Could you check a few things on this model? Use its own coordinates, in mm. A direction names the side the tool comes from. Round coordinates to 2 decimals unless told otherwise and drop trailing zeros. Loops run counter-clockwise (first coordinate to the right, second up) from the corner with the lowest first, then second, coordinate; pieces in that order, holes last. Notation, with made-up numbers: (16.25, 17) -> (65.25, 17) arc R11 cw to (65.25, 35) -> close; hole circle Ø5 at (6.5, 69). An arc over 180 degrees is marked (long way). One line per item, written item: value.
```python
from build123d import *
from build123d.topology import SkipClean

# Parameters (mm, degrees)
SKETCH1_R                            = 30
BOSS_EXTRUDE1_DEPTH                  = 4
BOSS_EXTRUDE2_REACH                  = 44.615
BOSS_EXTRUDE2_END_RADIUS             = 30
BOSS_EXTRUDE2_DIRECTION_2_REACH      = 44.615
BOSS_EXTRUDE2_DIRECTION_2_END_RADIUS = 30
SKETCH3_OUTSIDE_W                    = 78.092
SKETCH3_OUTSIDE_H                    = 69.092
SKETCH3_OUTSIDE_R                    = 21.5
CUT_EXTRUDE2_DEPTH                   = 12.5
BOSS_EXTRUDE3_DEPTH                  = 18
BOSS_EXTRUDE4_DEPTH                  = 15
BOSS_EXTRUDE5_DEPTH                  = 15
CUT_EXTRUDE3_DEPTH                   = 44.292609069
CUT_EXTRUDE3_DEPTH_BACK              = 44.292609069
SKETCH8_R                            = 2
CUT_EXTRUDE8_DEPTH                   = 48.077064479
CUT_EXTRUDE8_DEPTH_BACK              = 48.077064479
CUT_EXTRUDE9_DEPTH                   = 59.659818207
CUT_EXTRUDE11_DEPTH                  = 20
CUT_EXTRUDE12_DEPTH                  = 20
CUT_EXTRUDE13_DEPTH                  = 20
CUT_EXTRUDE14_DEPTH                  = 44.292609069
CUT_EXTRUDE14_DEPTH_BACK             = 44.292609069
SKETCH25_W                           = 66.075437062
SKETCH25_H                           = 20.142243048
SKETCH27_R                           = 1.375
CUT_EXTRUDE16_DEPTH                  = 30
SKETCH28_R                           = 5
CUT_EXTRUDE17_DEPTH                  = 3
CUT_EXTRUDE18_DEPTH                  = 43.690748412
CUT_EXTRUDE18_DEPTH_BACK             = 43.690748412
SKETCH29_W                           = 43.412566799
SKETCH29_H                           = 13.326200919
SKETCH32_W                           = 50
SKETCH32_H                           = 12
BOSS_EXTRUDE6_DEPTH                  = 18
SKETCH35_W                           = 12
SKETCH35_H                           = 15
BOSS_EXTRUDE7_DEPTH                  = 9
CUT_EXTRUDE19_DEPTH                  = 49.746794766
CUT_EXTRUDE19_DEPTH_BACK             = 49.746794766
SKETCH37_R                           = 2
SKETCH36_R                           = 2
CUT_EXTRUDE20_DEPTH                  = 15
SKETCH39_W                           = 12
SKETCH39_H                           = 15
BOSS_EXTRUDE8_DEPTH                  = 9
SKETCH40_R                           = 2
CUT_EXTRUDE21_DEPTH                  = 15
FILLET1_R                            = 3
FILLET2_R                            = 3
CUT_EXTRUDE24_START                  = -20
SKETCH44_R                           = 1.375
CUT_EXTRUDE24_DEPTH                  = 20
SKETCH45_R                           = 4.925
BOSS_EXTRUDE9_DEPTH                  = 42
SKETCH46_R                           = 1.8923
CUT_EXTRUDE25_DEPTH                  = 25.4
SKETCH47_R                           = 1.8923
CUT_EXTRUDE26_DEPTH                  = 25.4


with BuildPart() as part:
    # Sketch1 → Boss-Extrude1 (new body)
    with BuildSketch(Plane(origin=(0, 0, 0), x_dir=(1, 0, 0), z_dir=(0, 1, 0))):
        with Locations(Location((0, 0, 0), (0, 0, 270))):
            Circle(SKETCH1_R)
    extrude(amount=BOSS_EXTRUDE1_DEPTH)

    # Boss-Extrude2: up to this cylinder (the profile starts inside it)
    with SkipClean():  # the faces are left unmerged after this step: merging them gives an invalid solid
        boss_extrude2_end = Plane(origin=(0, 9.396175, 0), z_dir=(0, -1, 0)) * Cylinder(BOSS_EXTRUDE2_END_RADIUS, 150.23, mode=Mode.PRIVATE)
        # Sketch2 → Boss-Extrude2 (add, up to the surface)
        with BuildSketch(Plane(origin=(0, 0, 0), x_dir=(0, 0, -1), z_dir=(1, 0, 0)), mode=Mode.PRIVATE) as boss_extrude2_sk1:
            Polygon((0, 4), (21.5, 4), (9, 16.5), (-9, 16.5), (-21.5, 4), align=None)
        boss_extrude2_tool1 = extrude(boss_extrude2_sk1.sketch, amount=BOSS_EXTRUDE2_REACH, mode=Mode.PRIVATE) & boss_extrude2_end
        add(boss_extrude2_tool1.solids().sort_by_distance((0, 9.396175, 0))[0])

    # Boss-Extrude2 direction 2: up to this cylinder (the profile starts inside it)
    with SkipClean():  # the faces are left unmerged after this step: merging them gives an invalid solid
        boss_extrude2_direction_2_end = Plane(origin=(0, 9.396175, 0), z_dir=(0, -1, 0)) * Cylinder(BOSS_EXTRUDE2_DIRECTION_2_END_RADIUS, 150.23, mode=Mode.PRIVATE)
        # Sketch2 → Boss-Extrude2 direction 2 (add, up to the surface)
        with BuildSketch(Plane(origin=(0, 0, 0), x_dir=(0, 0, -1), z_dir=(1, 0, 0)), mode=Mode.PRIVATE) as boss_extrude2_direction_2_sk1:
            Polygon((0, 4), (21.5, 4), (9, 16.5), (-9, 16.5), (-21.5, 4), align=None)
        boss_extrude2_direction_2_tool1 = extrude(boss_extrude2_direction_2_sk1.sketch, amount=-BOSS_EXTRUDE2_DIRECTION_2_REACH, mode=Mode.PRIVATE) & boss_extrude2_direction_2_end
        add(boss_extrude2_direction_2_tool1.solids().sort_by_distance((0, 9.396175, 0))[0])

    # SurfaceCut1
    split(bisect_by=Plane(origin=(0, 12.75, -12.75), x_dir=(1, 0, 0), z_dir=(0, 0.7071067811865558, -0.7071067811865392)), keep=Keep.BOTTOM)

    # SurfaceCut2
    split(bisect_by=Plane(origin=(0, 12.75, 12.75), x_dir=(1, 0, 0), z_dir=(0, 0.7071067811865509, 0.7071067811865442)), keep=Keep.BOTTOM)

    # Sketch3 outside → Cut-Extrude2 (cut)
    with BuildSketch(Plane(origin=(0, 4, 0), x_dir=(1, 0, 0), z_dir=(0, 1, 0))):
        Rectangle(SKETCH3_OUTSIDE_W, SKETCH3_OUTSIDE_H)
        Circle(SKETCH3_OUTSIDE_R, mode=Mode.SUBTRACT)
    extrude(amount=CUT_EXTRUDE2_DEPTH, mode=Mode.SUBTRACT)

    # Sketch5 → Boss-Extrude3 (add)
    with BuildSketch(Plane(origin=(0, 0, 0), x_dir=(-1, 0, 0), z_dir=(0, -1, 0))):
        Polygon((0, -6), (-17.5, -6), (-17.5, 6), (17.5, 6), (17.5, -6), align=None)
    extrude(amount=BOSS_EXTRUDE3_DEPTH)

    # Sketch6 → Boss-Extrude4 (add)
    with BuildSketch(Plane.XZ):
        Polygon((0, 15), (7, 15), (7, 6), (-7, 6), (-7, 15), align=None)
    extrude(amount=BOSS_EXTRUDE4_DEPTH)

    # Sketch7 → Boss-Extrude5 (add)
    with BuildSketch(Plane.XZ):
        Polygon((0, -15), (7, -15), (7, -6), (-7, -6), (-7, -15), align=None)
    extrude(amount=BOSS_EXTRUDE5_DEPTH)

    # Sketch8 → Cut-Extrude3 (cut, two sides: drawn at the far end of the back side and taken through both)
    with BuildSketch(Plane.XY.offset(-CUT_EXTRUDE3_DEPTH_BACK)):
        with Locations((-12.5, -12.5)):
            Circle(SKETCH8_R)
        with Locations((12.5, -12.5)):
            Circle(SKETCH8_R)
    extrude(amount=CUT_EXTRUDE3_DEPTH + CUT_EXTRUDE3_DEPTH_BACK, mode=Mode.SUBTRACT)

    # Sketch16 → Cut-Extrude8 (cut, two sides: drawn at the far end of the back side and taken through both)
    with BuildSketch(Plane.XY.offset(6).offset(-CUT_EXTRUDE8_DEPTH_BACK)):
        Polygon((17.5, -18), (17.5, -14.5), (14, -18), align=None)
        Polygon((-17.5, -18), (-14, -18), (-17.5, -14.5), align=None)
    extrude(amount=CUT_EXTRUDE8_DEPTH + CUT_EXTRUDE8_DEPTH_BACK, mode=Mode.SUBTRACT)

    # Sketch17 → Cut-Extrude9 (cut, through all)
    with BuildSketch(Plane(origin=(10.365975269, -9.674910251, -8.062425209), x_dir=(-0.3613483622370374, 0.337258471421235, -0.8693009171531012), z_dir=(0.6355070151731325, -0.5931398808282571, -0.49428323402354774))):
        Polygon((-2.372510104, -6.189601271), (7.980636686, -0.706686759), (7.980636686, -10.965829024), align=None)
    extrude(amount=CUT_EXTRUDE9_DEPTH, mode=Mode.SUBTRACT)

    # Sketch19 → Cut-Extrude11 (cut)
    with BuildSketch(Plane(origin=(-10.365975269, -9.674910251, -8.062425209), x_dir=(0.3613483622370374, 0.33725847142123494, -0.8693009171531012), z_dir=(0.6355070151731324, 0.5931398808282571, 0.4942832340235476))):
        Polygon((-2.372510104, -6.189601271), (7.980636686, -10.965829024), (7.980636686, -0.706686759), align=None)
    extrude(amount=-CUT_EXTRUDE11_DEPTH, mode=Mode.SUBTRACT)

    # Sketch20 → Cut-Extrude12 (cut)
    with BuildSketch(Plane(origin=(-10.365975269, -9.674910251, 8.062425209), x_dir=(-0.3613483622370374, -0.3372584714212349, -0.8693009171531013), z_dir=(0.6355070151731326, 0.593139880828257, -0.49428323402354757))):
        Polygon((2.372510104, -6.189601271), (-7.980636686, -0.706686759), (-7.980636686, -10.965829024), align=None)
    extrude(amount=-CUT_EXTRUDE12_DEPTH, mode=Mode.SUBTRACT)

    # Sketch21 → Cut-Extrude13 (cut)
    with BuildSketch(Plane(origin=(10.365975269, -9.674910251, 8.062425209), x_dir=(-0.3613483622370374, 0.3372584714212349, 0.8693009171531013), z_dir=(-0.6355070151731326, 0.593139880828257, -0.49428323402354757))):
        Polygon((-2.372510104, -6.189601271), (7.980636686, -0.706686759), (7.980636686, -10.965829024), align=None)
    extrude(amount=-CUT_EXTRUDE13_DEPTH, mode=Mode.SUBTRACT)

    # Sketch25 → Cut-Extrude14 (cut, two sides: drawn at the far end of the back side and taken through both)
    with BuildSketch(Plane.XY.offset(-CUT_EXTRUDE14_DEPTH_BACK)):
        with Locations((0, -10.071121524)):
            Rectangle(SKETCH25_W, SKETCH25_H)
    extrude(amount=CUT_EXTRUDE14_DEPTH + CUT_EXTRUDE14_DEPTH_BACK, mode=Mode.SUBTRACT)

    # Sketch27 → Cut-Extrude16 (cut)
    with BuildSketch(Plane(origin=(0, 16.5, 0), x_dir=(1, 0, 0), z_dir=(0, 1, 0))):
        with Locations(Location((0, 0, 0), (0, 0, 270))):
            Circle(SKETCH27_R)
    extrude(amount=-CUT_EXTRUDE16_DEPTH, mode=Mode.SUBTRACT)

    # Sketch28 → Cut-Extrude17 (cut)
    with BuildSketch(Plane.XZ):
        with Locations(Location((0, -15, 0), (0, 0, 270))):
            Circle(SKETCH28_R)
        with Locations(Location((22, 0, 0), (0, 0, 270))):
            Circle(SKETCH28_R)
        with Locations(Location((0, 15, 0), (0, 0, 270))):
            Circle(SKETCH28_R)
        with Locations(Location((-22, 0, 0), (0, 0, 270))):
            Circle(SKETCH28_R)
        with Locations(Location((-14, 12, 0), (0, 0, 270))):
            Circle(SKETCH28_R)
        with Locations(Location((14, 12, 0), (0, 0, 270))):
            Circle(SKETCH28_R)
        with Locations(Location((14, -12, 0), (0, 0, 270))):
            Circle(SKETCH28_R)
        with Locations(Location((-14, -12, 0), (0, 0, 270))):
            Circle(SKETCH28_R)
    extrude(amount=-CUT_EXTRUDE17_DEPTH, mode=Mode.SUBTRACT)

    # Sketch29 → Cut-Extrude18 (cut, two sides: drawn at the far end of the back side and taken through both)
    with BuildSketch(Plane(origin=(0, 0, 0), x_dir=(0, 0, -1), z_dir=(1, 0, 0)).offset(-CUT_EXTRUDE18_DEPTH_BACK)):
        with Locations((0.2062834, 10.66310046)):
            Rectangle(SKETCH29_W, SKETCH29_H)
    extrude(amount=CUT_EXTRUDE18_DEPTH + CUT_EXTRUDE18_DEPTH_BACK, mode=Mode.SUBTRACT)

    # Sketch32 → Boss-Extrude6 (add)
    with BuildSketch(Plane(origin=(0, 4, 0), x_dir=(1, 0, 0), z_dir=(0, 1, 0))):
        Rectangle(SKETCH32_W, SKETCH32_H)
    extrude(amount=BOSS_EXTRUDE6_DEPTH)

    # Sketch35 → Boss-Extrude7 (add)
    with BuildSketch(Plane(origin=(0, 0, -6), x_dir=(-1, 0, 0), z_dir=(0, 0, -1))):
        with Locations((0, 11.5)):
            Rectangle(SKETCH35_W, SKETCH35_H)
    extrude(amount=BOSS_EXTRUDE7_DEPTH)

    # Sketch37 → Cut-Extrude19 (cut, two sides: drawn at the far end of the back side and taken through both)
    with BuildSketch(Plane(origin=(0, 0, -6), x_dir=(-1, 0, 0), z_dir=(0, 0, -1)).offset(-CUT_EXTRUDE19_DEPTH_BACK)):
        with Locations((-12.5, 18)):
            Circle(SKETCH37_R)
        with Locations((12.5, 18)):
            Circle(SKETCH37_R)
    extrude(amount=CUT_EXTRUDE19_DEPTH + CUT_EXTRUDE19_DEPTH_BACK, mode=Mode.SUBTRACT)

    # Sketch36 → Cut-Extrude20 (cut)
    with BuildSketch(Plane(origin=(0, 19, 0), x_dir=(1, 0, 0), z_dir=(0, 1, 0))):
        with Locations(Location((0, 10, 0), (0, 0, 270))):
            Circle(SKETCH36_R)
    extrude(amount=-CUT_EXTRUDE20_DEPTH, mode=Mode.SUBTRACT)

    # Sketch39 → Boss-Extrude8 (add)
    with BuildSketch(Plane.XY.offset(6)):
        with Locations((0, 11.5)):
            Rectangle(SKETCH39_W, SKETCH39_H)
    extrude(amount=BOSS_EXTRUDE8_DEPTH)

    # Sketch40 → Cut-Extrude21 (cut)
    with BuildSketch(Plane(origin=(0, 19, 0), x_dir=(1, 0, 0), z_dir=(0, 1, 0))):
        with Locations(Location((0, -10, 0), (0, 0, 270))):
            Circle(SKETCH40_R)
    extrude(amount=-CUT_EXTRUDE21_DEPTH, mode=Mode.SUBTRACT)

    # Fillet1
    fillet1_edges = [part.edges().sort_by_distance(p)[0] for p in [
        (25, 22, 0),
    ]]
    fillet(fillet1_edges, radius=FILLET1_R)

    # Fillet2
    fillet2_edges = [part.edges().sort_by_distance(p)[0] for p in [
        (-25, 22, 0),
    ]]
    fillet(fillet2_edges, radius=FILLET2_R)

    # Sketch44 → Cut-Extrude24 (cut)
    with BuildSketch(Plane.XZ.offset(-4).offset(CUT_EXTRUDE24_START)):
        with Locations(Location((0, 0, 0), (0, 0, 90))):
            Circle(SKETCH44_R)
    extrude(amount=CUT_EXTRUDE24_DEPTH, mode=Mode.SUBTRACT)

    # Sketch45 → Boss-Extrude9 (add)
    with BuildSketch(Plane.XZ):
        with Locations(Location((-8, 0, 0), (0, 0, 90))):
            Circle(SKETCH45_R)
        with Locations(Location((8, 0, 0), (0, 0, 90))):
            Circle(SKETCH45_R)
    extrude(amount=BOSS_EXTRUDE9_DEPTH)

    # Sketch46 → Cut-Extrude25 (cut)
    with BuildSketch(Plane.XZ.offset(42)):
        with Locations(Location((-8, 0, 0), (0, 0, 270))):
            Circle(SKETCH46_R)
    extrude(amount=-CUT_EXTRUDE25_DEPTH, mode=Mode.SUBTRACT)

    # Sketch47 → Cut-Extrude26 (cut)
    with BuildSketch(Plane.XZ.offset(42)):
        with Locations(Location((8, 0, 0), (0, 0, 270))):
            Circle(SKETCH47_R)
    extrude(amount=-CUT_EXTRUDE26_DEPTH, mode=Mode.SUBTRACT)


solid = part.part
```
(1) Imagine slicing it at C-C on x = 8. Write out the boundary of the cut face in (y, z) (3 decimals).
Results below:
outline: (-42, -4.925) -> (0, -4.925) -> (0, -25.5) -> (4, -21.5) -> (4, -6) -> (22, -6) -> (22, 6) -> (4, 6) -> (4, 21.5) -> (0, 25.5) -> (0, 4.925) -> (-42, 4.925) -> (-42, 1.892) -> (-16.6, 1.892) -> (-16.6, -1.892) -> (-42, -1.892) -> close
(2) Imagine slicing it at B-B on y = -26. Write out the boundary of the cut face in (x, z) (3 decimals).
Results below:
outline: circle Ø9.85 at (-8, 0); circle Ø9.85 at (8, 0); hole circle Ø3.785 at (-8, 0); hole circle Ø3.785 at (8, 0)
(3) Imagine slicing it at A-A on y = 17. Write out the boundary of the cut face in (x, z) (3 decimals), then the cut area to 3 significant figures.
Results below:
outline: (-25, -6) -> (-14.232, -6) -> (-14.232, 6) -> (-25, 6) -> close; (-10.768, -6) -> (-6, -6) -> (-6, -15) -> (6, -15) -> (6, -6) -> (10.768, -6) -> (10.768, 6) -> (6, 6) -> (6, 15) -> (-6, 15) -> (-6, 6) -> (-10.768, 6) -> close; (14.232, -6) -> (25, -6) -> (25, 6) -> (14.232, 6) -> close; hole circle Ø4 at (0, -10); hole circle Ø4 at (0, 10); hole circle Ø2.75 at (0, 0)
area: 702 mm²
(4) Please list where these lines run through material, in increasing order: L1, parallel to X at y = 2, z = 0 (3 decimals); L2, parallel to X at y = 2.45, z = 12; L3, parallel to X at y = -23.5, z = -4.
Results below:
L1: x = -30 to -27, -17 to -1.375, 1.375 to 17, 27 to 30
L2: x = -27.5 to -19, -9 to -4, 4 to 9, 19 to 27.5
L3: x = -10.87 to -5.13, 5.13 to 10.87
(5) For pin 1 Ø3 at (x, z) = (-13, 11) entering from -Y; pin 2 Ø6 at (x, y) = (-2.5, 10.5) entering from +Z; pin 3 Ø4 at (x, z) = (-18, -9.5) entering from +Y, each with a flat end and sliding along its axis, tell me the tip position at first contact or that it passes through.
Results below:
pin 1: stops at y = 3
pin 2: stops at z = 15
pin 3: stops at y = 4
(6) Imagine slicing it at D-D on y = -15.5. Write out the boundary of the cut face in (x, z) (3 decimals), then the cut area to 3 significant figures.
Results below:
outline: circle Ø9.85 at (-8, 0); circle Ø9.85 at (8, 0)
area: 152 mm²
(7) On a 3-axis mill with a long thin cutter (end or side, diameter ignored), from which of +Z, -Z, +X, -X, +Y, -Y can I reach the whole of each face in a straight line? I mean faces 1 (the face through (6, 11, -10)), 2 (the face through (0, 4, 10)), 3 (the face through (0.1, 19, -12.4)). Say none if no direction works.
Results below:
face 1: -Z, +X, +Y
face 2: +Y
face 3: -Z, +X, -X, +Y
